The drawing under review shows one solid part. Ordinate dimensions are in mm from its lowest x, y, z. A direction names the side the tool comes from. Round coordinates to 2 decimals unless told otherwise and drop trailing zeros. Order: outer loops, then holes, each group sorted by start corner. A loop starts at its lowest first (then second) coordinate and runs counter-clockwise, first axis right, second up. Notation, with made-up numbers: (61.25, 64.5) -> (100.25, 64.5) arc R20 ccw to (100.25, 92.5) -> close; hole circle Ø8 at (45, 35.25). An arc over 180 degrees is marked (long way). Put each result on its own line as item: value. Start each with the question number.
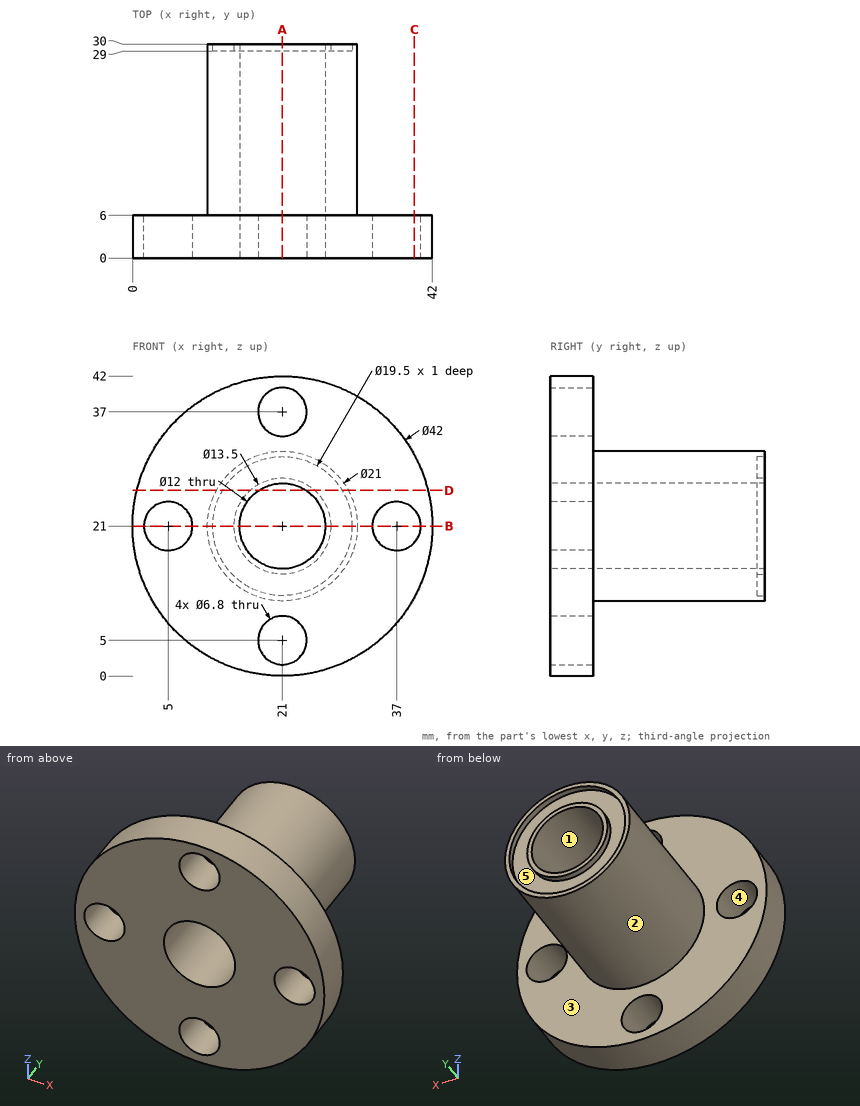
Item 1: Mouldability with a two-part tool opening along Z and no side actions: class the marked faces 1, 2 and 3 as +Z half, -Z half, draft (parallel to the pull), parting line (faces both ways), or undercut.
Item 2: Consider section D-D, the plane z = 26. Write out the cut boundary in (x, y).
Item 3: Tool access review of the marked faces 4 and 5: name each direction out of +Z, -Z, +X, -X, +Y, -Y from which nothing blocks a thin tool from reaching the whole face with its end or side.
Item 4: Insertion check: pin 1 Ø5.5 at (x, z) = (21, 37) entering from -Y; pin 2 Ø4 at (y, z) = (15.5, 24) entering from -X; pin 3 Ø1 at (x, y) = (22, 27) entering from +Z; pin 4 Ø2 at (x, y) = (10.5, 15) entering from +Z. Each pin has a flat end and moves straight along its axis. Give the tip position at first contact, or say it passes through.
Item 5: Consider section C-C, the plane x = 39.5. Write out the cut boundary in (y, z).
Item 6: For L1, parallel to X at y = 28.5, z = 21; L2, parallel to Y at x = 10.5, z = 7.5; L3, parallel to Z at x = 37, y = 2, list the stretches that pass through material, from the lowest coordinate up.
Item 7: Consider section A-A, the plane x = 21. Write out the cut boundary in (y, z).
Item 8: Consider section B-B, the plane z = 21. Write out the cut boundary in (x, y), plus the area to 3 significant figures.
Evaluation:
1. face 1: undercut
1. face 2: parting line
1. face 3: draft
2. outline: (0.6, 0) -> (17.68, 0) -> (17.68, 30) -> (16.47, 30) -> (16.47, 29) -> (12.63, 29) -> (12.63, 30) -> (11.77, 30) -> (11.77, 6) -> (0.6, 6) -> close; (24.32, 0) -> (41.4, 0) -> (41.4, 6) -> (30.23, 6) -> (30.23, 30) -> (29.37, 30) -> (29.37, 29) -> (25.53, 29) -> (25.53, 30) -> (24.32, 30) -> close
3. face 4: +Y, -Y
3. face 5: +Y
4. pin 1: passes through
4. pin 2: stops at x = 10.55
4. pin 3: stops at z = 31.49
4. pin 4: stops at z = 25.47
5. outline: (0, 11.06) -> (6, 11.06) -> (6, 18.7) -> (0, 18.7) -> close; (0, 23.3) -> (6, 23.3) -> (6, 30.94) -> (0, 30.94) -> close
6. L1: x = 10.5 to 15, 27 to 31.5
6. L2: y = 0 to 6
6. L3: z = 7.4 to 17.6, 24.4 to 34.6
7. outline: (0, 0) -> (6, 0) -> (6, 1.6) -> (0, 1.6) -> close; (0, 8.4) -> (6, 8.4) -> (6, 10.5) -> (30, 10.5) -> (30, 11.25) -> (29, 11.25) -> (29, 14.25) -> (30, 14.25) -> (30, 15) -> (0, 15) -> close; (0, 27) -> (30, 27) -> (30, 27.75) -> (29, 27.75) -> (29, 30.75) -> (30, 30.75) -> (30, 31.5) -> (6, 31.5) -> (6, 33.6) -> (0, 33.6) -> close; (0, 40.4) -> (6, 40.4) -> (6, 42) -> (0, 42) -> close
8. outline: (0, 0) -> (1.6, 0) -> (1.6, 6) -> (0, 6) -> close; (8.4, 0) -> (15, 0) -> (15, 30) -> (14.25, 30) -> (14.25, 29) -> (11.25, 29) -> (11.25, 30) -> (10.5, 30) -> (10.5, 6) -> (8.4, 6) -> close; (27, 0) -> (33.6, 0) -> (33.6, 6) -> (31.5, 6) -> (31.5, 30) -> (30.75, 30) -> (30.75, 29) -> (27.75, 29) -> (27.75, 30) -> (27, 30) -> close; (40.4, 0) -> (42, 0) -> (42, 6) -> (40.4, 6) -> close
8. area: 308 mm^2
